Can you work these out from the model? Positions are in its coordinate system, mm. Face numbers are marked on the shaded views. Give positions to 0.01 mm unless a question says otherwise; leave off trailing zeros. Write each loop counter-clockwise with the first axis right and the second up, starting at its lowest first coordinate (ties: lowest second). Pieces come first, ordered by that corner, then holes. Notation, with made-up numbers: (79, -30.5) -> (111, -30.5) arc R22 ccw to (111, 1.5) -> close; hole circle Ø10 at (-27, 27.5). An arc over 180 degrees is marked (long way). Answer as CSV lines item,"result". Start each with the question number.
1. If we section it at B-B on x = 6: Write out the boundary of the cut face in (y, z), plus the area to 3 significant figures.
2. I'm going to push flat-ended pins straight in: P1, Ø7, axis at x = 20.75, y = 0, coming from the -Z side; P2, Ø8, axis at x = 10.38, y = 17.97, coming from the +Z side; P3, Ø5, axis at x = 0, y = 20.75, coming from the -Z side; P4, Ø2, axis at x = 8, z = 0, coming from the -Y side. Where does each tip first touch, or does it pass through?
3. If we mould it in two halves opening along Y, with no side actions, what happens to the marked faces 1, 2 and 3? For each: pulls with the +Y half, pulls with the -Y half, needs draft (parallel to the pull), parting line crosses it, or undercut.
4. If we section it at D-D on x = -23: Write out the boundary of the cut face in (y, z), plus the area to 3 significant figures.
5. I need wall thicknesses on line 1 (Y direction, x = 20.5, z = 0.3); line 2 (Y direction, x = 0, z = 0.35) (3 decimals); line 3 (Z direction, x = -2, y = 24.5). Which ranges of each line are inside material? Lowest first, please. Write a range as [from, to].
6. If we section it at A-A on x = 0: Count the separate pieces of the cut face and the enclosed holes in it, plus the area to 3 significant figures.
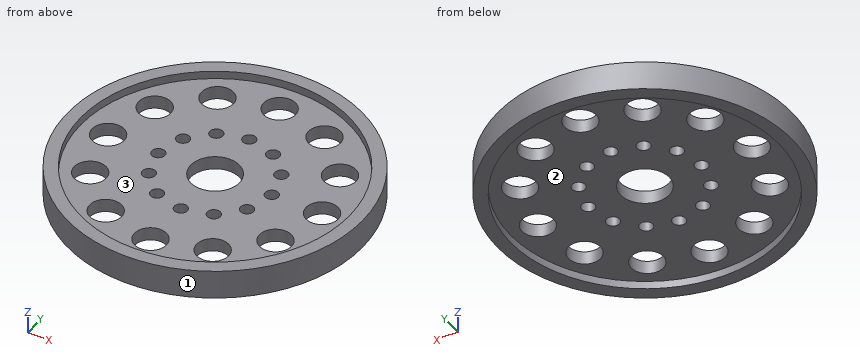
```python
from build123d import *

# Parameters (mm, degrees)
SKETCH1_R               = 28.575
BOSS_EXTRUDE1_DEPTH     = 2.794
SKETCH2_R               = 4.71805
SKETCH2_R_2             = 1.27
CUT_EXTRUDE1_DEPTH      = 41.795673717
CUT_EXTRUDE2_START      = -1.27
SKETCH3_R               = 26.035
CUT_EXTRUDE2_DEPTH      = 1.651
CUT_EXTRUDE3_DEPTH      = 41.507625035
CUT_EXTRUDE3_DEPTH_BACK = 41.507625035
SKETCH4_R               = 3.10515


with BuildPart() as part:
    # Sketch1 → Boss-Extrude1 (new, symmetric)
    with BuildSketch(Plane.XY):
        Circle(SKETCH1_R)
    extrude(amount=BOSS_EXTRUDE1_DEPTH, both=True)

    # Sketch2 → Cut-Extrude1 (cut, through all)
    with BuildSketch(Plane.XY.offset(2.794)):
        Circle(SKETCH2_R)
        with Locations((0, 11)):
            Circle(SKETCH2_R_2)
        with Locations((5.500133975, 9.526779442)):
            Circle(SKETCH2_R_2)
        with Locations((9.526779442, 5.500866025)):
            Circle(SKETCH2_R_2)
        with Locations((11.001, 0.001)):
            Circle(SKETCH2_R_2)
        with Locations((9.527779442, -5.499133975)):
            Circle(SKETCH2_R_2)
        with Locations((5.501866025, -9.525779442)):
            Circle(SKETCH2_R_2)
        with Locations((0.002, -11)):
            Circle(SKETCH2_R_2)
        with Locations((-5.498133975, -9.526779442)):
            Circle(SKETCH2_R_2)
        with Locations((-9.524779442, -5.500866025)):
            Circle(SKETCH2_R_2)
        with Locations((-10.999, -0.001)):
            Circle(SKETCH2_R_2)
        with Locations((-9.525779442, 5.499133975)):
            Circle(SKETCH2_R_2)
        with Locations((-5.499866025, 9.525779442)):
            Circle(SKETCH2_R_2)
    extrude(amount=-CUT_EXTRUDE1_DEPTH, mode=Mode.SUBTRACT)

    # Sketch3 → Cut-Extrude2 (cut)
    with BuildSketch(Plane.XY.offset(CUT_EXTRUDE2_START)):
        Circle(SKETCH3_R)
    cut_extrude2 = extrude(amount=-CUT_EXTRUDE2_DEPTH, mode=Mode.SUBTRACT)

    # Mirror1: Cut-Extrude2 across plane
    add(cut_extrude2.mirror(Plane.XY), mode=Mode.SUBTRACT)

    # Sketch4 → Cut-Extrude3 (cut, two sides: drawn at the far end of the back side and taken through both)
    with BuildSketch(Plane.XY.offset(-CUT_EXTRUDE3_DEPTH_BACK)):
        with Locations((0, 20.75)):
            Circle(SKETCH4_R)
        with Locations((10.375, 17.970027129)):
            Circle(SKETCH4_R)
        with Locations((17.970027129, 10.375)):
            Circle(SKETCH4_R)
        with Locations((20.75, 0)):
            Circle(SKETCH4_R)
        with Locations((17.970027129, -10.375)):
            Circle(SKETCH4_R)
        with Locations((10.375, -17.970027129)):
            Circle(SKETCH4_R)
        with Locations((0, -20.75)):
            Circle(SKETCH4_R)
        with Locations((-10.375, -17.970027129)):
            Circle(SKETCH4_R)
        with Locations((-17.970027129, -10.375)):
            Circle(SKETCH4_R)
        with Locations((-20.75, 0)):
            Circle(SKETCH4_R)
        with Locations((-17.970027129, 10.375)):
            Circle(SKETCH4_R)
        with Locations((-10.375, 17.970027129)):
            Circle(SKETCH4_R)
    extrude(amount=CUT_EXTRUDE3_DEPTH + CUT_EXTRUDE3_DEPTH_BACK, mode=Mode.SUBTRACT)


solid = part.part
```
Computed values:
1,outline,"(-27.94, -2.79) -> (-25.33, -2.79) -> (-25.33, -1.27) -> (-10.69, -1.27) -> (-10.69, 1.27) -> (-25.33, 1.27) -> (-25.33, 2.79) -> (-27.94, 2.79) -> close; (-8.36, -1.27) -> (8.36, -1.27) -> (8.36, 1.27) -> (-8.36, 1.27) -> close; (10.69, -1.27) -> (25.33, -1.27) -> (25.33, -2.79) -> (27.94, -2.79) -> (27.94, 2.79) -> (25.33, 2.79) -> (25.33, 1.27) -> (10.69, 1.27) -> close"
1,area,"146 mm2"
2,P1,"stops at z = -1.27"
2,P2,"stops at z = 1.27"
2,P3,"passes through"
2,P4,"stops at y = -27.7"
3,face 1,"parting line crosses it"
3,face 2,"undercut"
3,face 3,"undercut"
4,outline,"(-16.96, -2.79) -> (-12.2, -2.79) -> (-12.2, -1.27) -> (-2.14, -1.27) -> (-2.14, 1.27) -> (-12.2, 1.27) -> (-12.2, 2.79) -> (-16.96, 2.79) -> close; (2.14, -1.27) -> (12.2, -1.27) -> (12.2, -2.79) -> (16.96, -2.79) -> (16.96, 2.79) -> (12.2, 2.79) -> (12.2, 1.27) -> (2.14, 1.27) -> close"
4,area,"104 mm2"
5,line 1,"y = [-19.91, -12.18], [-8.57, -3.1], [3.1, 8.57], [12.18, 19.91]"
5,line 2,"y = [-28.575, -23.855], [-17.645, -12.27], [-9.73, -4.718], [4.718, 9.73], [12.27, 17.645], [23.855, 28.575]"
5,line 3,"z = [-1.27, 1.27]"
6,separate pieces,"6"
6,enclosed holes,"0"
6,area,"92.2 mm2"
